```python
from build123d import *

# Parameters (mm, degrees)
SKETCH1_R               = 300
SKETCH1_R_2             = 225
BOSS_EXTRUDE1_DEPTH     = 20
SKETCH1_R_3             = 90
BOSS_EXTRUDE1_2_DEPTH   = 20
SKETCH3_R               = 225
BOSS_EXTRUDE3_DEPTH     = 5
CHAMFER2_SIZE           = 15
CUT_EXTRUDE1_DEPTH      = 425.735211632
CUT_EXTRUDE1_DEPTH_BACK = 425.735211632
SKETCH4_R               = 22.5


with BuildPart() as part:
    # Sketch1 → Boss-Extrude1 (new, symmetric)
    with BuildSketch(Plane(origin=(0, 0, 0), x_dir=(1, 0, 0), z_dir=(0, 1, 0))):
        with Locations(Location((0, 0, 0), (0, 0, 270))):
            Circle(SKETCH1_R)
        with Locations(Location((0, 0, 0), (0, 0, 270))):
            Circle(SKETCH1_R_2, mode=Mode.SUBTRACT)
    extrude(amount=BOSS_EXTRUDE1_DEPTH, both=True)



with BuildPart() as body_2:
    # Sketch1 → Boss-Extrude1 2 (new, symmetric)
    with BuildSketch(Plane(origin=(0, 0, 0), x_dir=(1, 0, 0), z_dir=(0, 1, 0))):
        with Locations(Location((0, 0, 0), (0, 0, 270))):
            Circle(SKETCH1_R_3)
    extrude(amount=BOSS_EXTRUDE1_2_DEPTH, both=True)


with BuildPart() as part_1:
    add(part.part)

    add(body_2.part)  # Boss-Extrude3 merges body 2
    # Sketch3 → Boss-Extrude3 (add, symmetric)
    with BuildSketch(Plane(origin=(0, 0, 0), x_dir=(1, 0, 0), z_dir=(0, 1, 0))):
        with Locations(Location((0, 0, 0), (0, 0, 270))):
            Circle(SKETCH3_R)
    extrude(amount=BOSS_EXTRUDE3_DEPTH, both=True)

    # Chamfer2
    chamfer2_edges = [part_1.edges().sort_by_distance(p)[0] for p in [
        (0, -20, -90),
        (0, 20, -90),
        (0, -20, -225),
        (0, 20, -225),
    ]]
    chamfer(chamfer2_edges, length=CHAMFER2_SIZE - 0.0001)  # a hair under: the kernel refuses the full size

    # Sketch4 → Cut-Extrude1 (cut, two sides: drawn at the far end of the back side and taken through both)
    with BuildSketch(Plane(origin=(0, 0, 0), x_dir=(1, 0, 0), z_dir=(0, 1, 0)).offset(-CUT_EXTRUDE1_DEPTH_BACK)):
        with Locations(Location((0, 0, 0), (0, 0, 270))):
            Circle(SKETCH4_R)
        with Locations(Location((-110, 110, 0), (0, 0, 270))):
            Circle(SKETCH4_R)
        with Locations(Location((110, 110, 0), (0, 0, 270))):
            Circle(SKETCH4_R)
        with Locations(Location((110, -110, 0), (0, 0, 270))):
            Circle(SKETCH4_R)
        with Locations(Location((-110, -110, 0), (0, 0, 270))):
            Circle(SKETCH4_R)
    extrude(amount=CUT_EXTRUDE1_DEPTH + CUT_EXTRUDE1_DEPTH_BACK, mode=Mode.SUBTRACT)


solid = part_1.part
```
Verification items for the finished model (mm, model axes). A direction names the side the tool comes from. Coordinates: 2 decimals unless noted, no trailing zeros. Order: outer loops, then holes, each group sorted by start corner. A loop starts at its lowest first (then second) coordinate and runs counter-clockwise, first axis right, second up. Notation, with made-up numbers: (56, -5) - (115, -5) arc R19 ccw to (115, 29) - close; hole circle Ø5 at (83, 4). An arc over 180 degrees is marked (long way). Return JSON: item names as keys, results as strings.
(1) Mould release check, pull along Z, two halves, no side actions. Record for faces 4 (the conical face through (67.866, -5.938, 215.505)), 5 (the flat face through (201, -20, -135)), 6 (the cylindrical face through (-182.545, 0.28, -238.07)): pulls with the +Z half, pulls with the -Z half, needs draft (parallel to the pull), parting line crosses it, or undercut.
Filled sheet:
{"face 4": "undercut", "face 5": "needs draft", "face 6": "parting line crosses it"}
(2) Go/stop test with flat-tipped pins: pin 1 (3 mm diameter, centred on y = -11, z = 115.5, fed in from -X); pin 2 (10 mm diameter, centred on x = -176.5, y = 4.5, fed in from -Z); pin 3 (1 mm diameter, centred on y = 14.5, z = -230, fed in from +X). Record where each tip stops, or that it passes through.
Filled sheet:
{"pin 1": "stops at x = -277.5", "pin 2": "stops at z = -246.15", "pin 3": "stops at x = 193.21"}
(3) Access from +Z, -Z, +X, -X, +Y, -Y to the whole of each face (thin tool, end or side, straight path). Record for faces 1 (the flat face through (3, -5, 97)), 2 (the flat face through (3, 5, 97)), 3 (the cylindrical face through (-8.618, -0.28, 20.784)).
Filled sheet:
{"face 1": "-Y", "face 2": "+Y", "face 3": "+Y, -Y"}
(4) Section check C-C, the plane x = 110. Give the number of separate pieces and of enclosed holes in the cut face, and give its area (3 significant figures).
Filled sheet:
{"separate pieces": "3", "enclosed holes": "0", "area": "9,140 mm^2"}
(5) Section check B-B, the plane y = 11.5. Record the cut outline in (x, z).
Filled sheet:
{"outline": "circle Ø600 at (0, 0); circle Ø167 at (0, 0); hole circle Ø463 at (0, 0); hole circle Ø45 at (0, 0)"}
(6) Thickness scan on line 1 along Z through (x, y) = (-110, 2); line 2 along X through (y, z) = (4, 0); line 3 along X through (y, z) = (-14, -50). Record the ranges inside material, lowest first.
Filled sheet:
{"line 1": "z = -279.11 to -132.5, -87.5 to 87.5, 132.5 to 279.11", "line 2": "x = -300 to -22.5, 22.5 to 300", "line 3": "x = -295.8 to -228.6, -63.73 to 63.73, 228.6 to 295.8"}
